Can you work these out from the drawing? Everything is in mm from the part's minimum corner. A direction names the side the tool comes from. Give positions to 0.01 mm unless a question says otherwise; leave off trailing zeros. Order: outer loops, then holes, each group sorted by start corner. A loop starts at its lowest first (then second) coordinate and runs counter-clockwise, first axis right, second up. Notation, with made-up numbers: M -17,25 L -4,25 A10 ccw -4,38 Z; hole C 61.25,76 d2. An arc over 180 degrees is marked long. Use a Markdown table: item, result. Add a question column.
Item 1: For the marked faces 1 and 2, which set-ups out of +Z, -Z, +X, -X, +Y, -Y let a thin tool reach every point of the face, with its end or its side?
Item 2: Suppose I cut it at B-B on z = 12.7. Write out the boundary of the cut face in (x, y).
Item 3: Suppose I cut it at C-C on y = 69.85. Write out the boundary of the cut face in (x, z).
Item 4: If we mould it in two halves opening along Y, with no side actions, what happens to the marked faces 3, 4 and 5? For each: released by +Y, released by -Y, zero draft, split by the parting line, or undercut.
Item 5: If I drill on L1, parallel to Y at x = 6.75, z = 12.7; L2, parallel to Y at x = 6.35, z = 6.5; L3, parallel to Y at x = 6.5, z = 15.5, over which ranges is the centre line in solid material (lowest first)? Write a range as from..to.
Item 6: I'm going to push flat-ended pins straight in: pin 1 Ø3 at (x, y) = (6.35, 5.08) entering from -Z; pin 2 Ø1 at (y, z) = (30, 10) entering from +X. Where does each tip first touch, or does it pass through?
Item 7: Suppose I cut it at A-A on x = 9.5. Count the separate pieces of the cut face and the enclosed holes in it, plus the area to 3 significant figures.
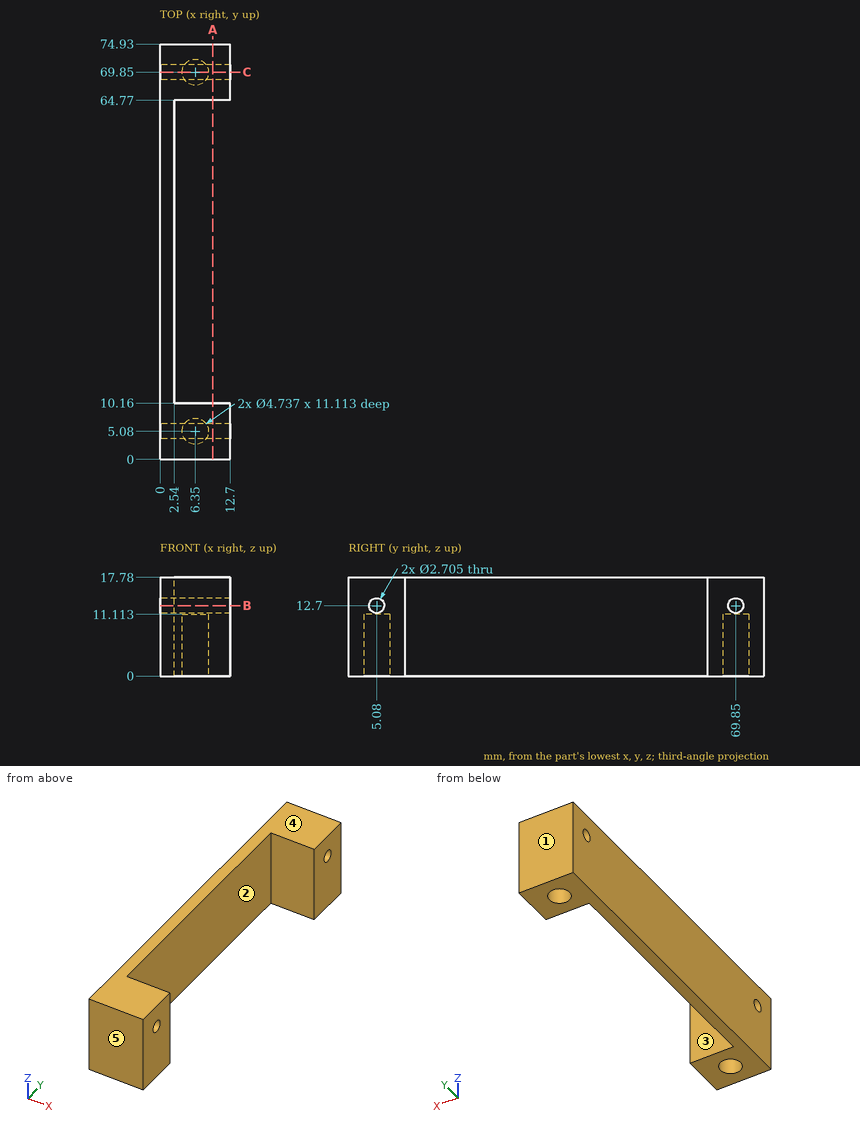
Findings below:
| question | item | result |
|---|---|---|
| 1 | face 1 | +Z, -Z, +X, -X, +Y |
| 1 | face 2 | +Z, -Z, +X |
| 2 | outline | M 0,0 L 12.7,0 L 12.7,3.73 L 0,3.73 Z; M 0,6.43 L 12.7,6.43 L 12.7,10.16 L 2.54,10.16 L 2.54,64.77 L 12.7,64.77 L 12.7,68.5 L 0,68.5 Z; M 0,71.2 L 12.7,71.2 L 12.7,74.93 L 0,74.93 Z |
| 3 | outline | M 0,0 L 3.98,0 L 3.98,11.11 L 8.72,11.11 L 8.72,0 L 12.7,0 L 12.7,11.35 L 0,11.35 Z; M 0,14.05 L 12.7,14.05 L 12.7,17.78 L 0,17.78 Z |
| 4 | face 3 | undercut |
| 4 | face 4 | zero draft |
| 4 | face 5 | released by -Y |
| 5 | L1 | y = 0..3.73, 6.43..10.16, 64.77..68.5, 71.2..74.93 |
| 5 | L2 | y = 0..2.71, 7.45..10.16, 64.77..67.48, 72.22..74.93 |
| 5 | L3 | y = 0..10.16, 64.77..74.93 |
| 6 | pin 1 | stops at z = 11.11 |
| 6 | pin 2 | stops at x = 2.54 |
| 7 | separate pieces | 2 |
| 7 | enclosed holes | 2 |
| 7 | area | 350 mm^2 |
